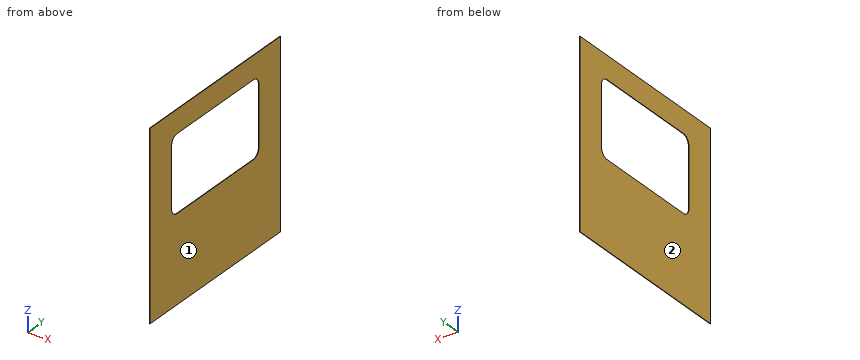
```python
from build123d import *

# Parameters (mm, degrees)
F0_W     = 1200
F0_H     = 1200
F1_DEPTH = 3


with BuildPart() as f1:
    # F0 (on Right) → F1 (new body)
    with BuildSketch(Plane.YZ):
        with Locations((-365.502932, 10.141731)):
            Rectangle(F0_W, F0_H)
        with BuildLine():
            ThreePointArc((-765.502932, 410.141731), (-750.858271, 445.49707), (-715.502932, 460.141731))
            Line((-715.502932, 460.141731), (-15.502932, 460.141731))
            ThreePointArc((-15.502932, 460.141731), (19.852408, 445.49707), (34.497068, 410.141731))
            Line((34.497068, 410.141731), (34.497068, 20.141731))
            ThreePointArc((34.497068, 20.141731), (19.852408, -15.213608), (-15.502932, -29.858269))
            Line((-15.502932, -29.858269), (-715.502932, -29.858269))
            ThreePointArc((-715.502932, -29.858269), (-750.858271, -15.213608), (-765.502932, 20.141731))
            Line((-765.502932, 20.141731), (-765.502932, 410.141731))
        make_face(mode=Mode.SUBTRACT)
    extrude(amount=-F1_DEPTH)


solid = f1.part
```
Could you check a few things on this model? Use its own coordinates, in mm. Face numbers are marked on the shaded views. Round coordinates to 2 decimals unless told otherwise and drop trailing zeros. Loops run counter-clockwise (first coordinate to the right, second up) from the corner with the lowest first, then second, coordinate; pieces in that order, holes last. Notation, with made-up numbers: (-9, 24.5) - (10, 24.5) arc R16 ccw to (10, 40.5) - close; hole circle Ø11 at (27, 45.25). An arc over 180 degrees is marked (long way). Answer in a Markdown table with one row per item. Add a question column.
(1) If we section it at C-C (x = -2.4): Please give me the cut outline in (y, z), plus the area to 3 significant figures.
(2) If we section it at A-A (y = -680): Please give me the cut outline in (x, z).
(3) I'm going to push a flat-ended pin straight in: pin 1 (1.5 mm diameter, centred on y = -633, z = -374.5, fed in from +X). Where does the tip first touch, or does it pass through?
(4) If we section it at B-B (z = 150): Please give me the cut outline in (x, y), plus the area to 3 significant figures.
(5) I need wall thicknesses on line 1 along Y through (x, z) = (-0.35, 307); line 2 along Z through (x, y) = (-2.35, -379.5); line 3 along Z through (x, y) = (-1.95, -9). Which ranges of each line are inside material? Lowest first, please.
(6) If we mould it in two halves opening along X, with no side actions, what happens to the marked faces 1 and 2? For each: pulls with the +X half, pulls with the -X half, needs draft (parallel to the pull), parting line crosses it, or undercut.
Model answer:
| question | item | result |
|---|---|---|
| 1 | outline | (-965.5, -589.86) - (234.5, -589.86) - (234.5, 610.14) - (-965.5, 610.14) - close; hole (-765.5, 20.14) arc R50 ccw to (-715.5, -29.86) - (-15.5, -29.86) arc R50 ccw to (34.5, 20.14) - (34.5, 410.14) arc R50 ccw to (-15.5, 460.14) - (-715.5, 460.14) arc R50 ccw to (-765.5, 410.14) - close |
| 1 | area | 1,050,000 mm² |
| 2 | outline | (-3, -589.86) - (0, -589.86) - (0, -29.86) - (-3, -29.86) - close; (-3, 460.14) - (0, 460.14) - (0, 610.14) - (-3, 610.14) - close |
| 3 | pin 1 | stops at x = 0 |
| 4 | outline | (-3, -965.5) - (0, -965.5) - (0, -765.5) - (-3, -765.5) - close; (-3, 34.5) - (0, 34.5) - (0, 234.5) - (-3, 234.5) - close |
| 4 | area | 1,200 mm² |
| 5 | line 1 | y = -965.5 to -765.5, 34.5 to 234.5 |
| 5 | line 2 | z = -589.86 to -29.86, 460.14 to 610.14 |
| 5 | line 3 | z = -589.86 to -29.43, 459.72 to 610.14 |
| 6 | face 1 | pulls with the +X half |
| 6 | face 2 | pulls with the -X half |
